Source: CAD feature listing. Evaluate the final solid. Frame: model axes, mm. A direction names the side the tool comes from. Round coordinates to 2 decimals unless told otherwise and drop trailing zeros. Loops run counter-clockwise (first coordinate to the right, second up) from the corner with the lowest first, then second, coordinate; pieces in that order, holes last. Notation, with made-up numbers: (-26, 19) - (-6, 19) arc R20 ccw to (-6, 51) - close; hole circle Ø2 at (88.5, 52.25). An arc over 180 degrees is marked (long way). One line per question, with ' | ' between items. Start each with the question number.
1. Cut plane A-A (x = 0). Return loops of the section in (y, z), then the cut area to 3 significant figures.
2. Pin query (flat end, axial travel): pin 1 (3 mm diameter, centred on x = -8.5, y = 35.5, fed in from +Z); pin 2 (1 mm diameter, centred on x = 0, y = 33, fed in from +Z); pin 3 (1.5 mm diameter, centred on x = 13, y = 9.5, fed in from +Z). Return the tip coordinate at first contact, or that it passes through.
3. Cut plane B-B (z = 19). Return loops of the section in (x, y), then the cut area to 3 significant figures.
4. Access query for faces 4 (the flat face through (9, 40, 39)), 5 (the flat face through (0, 48, 50)), 6 (the flat face through (5, 20, 10)). Directions: +Z, -Z, +X, -X, +Y, -Y. A direction counts if a zero-diameter tool reaches every point of the face in a straight line with its end or side. Return the directions, or none.
5. Cut plane D-D (z = 14). Return loops of the section in (x, y), then the cut area to 3 significant figures.
6. Cut plane C-C (y = 16). Return loops of the section in (x, z), then the cut area to 3 significant figures.
7. Ray query, line 1 (X direction, y = 26, z = 40); line 2 (Y direction, x = -6.5, z = 33.5); line 3 (Y direction, x = -3.5, z = 21.5). Return the intervals inside material, ascending.
8. Mould query, pull axis Y, two halves, no side actions, for faces 1 (the flat face through (-10, 20, 25)), 2 (the flat face through (-5, 6, 35)), 3 (the flat face through (-5, 0, 19)). Classes: pulls with the +Y half, pulls with the -Y half, needs draft (parallel to the pull), parting line crosses it, or undercut.
```python
from build123d import *

# Parameters (mm, degrees)
F1_DEPTH = 50
F3_W     = 30
F3_H     = 20
F4_DEPTH = 40
F5_DEPTH = 40


with BuildPart() as f1:
    # F0 (on Top) → F1 (new body)
    with BuildSketch(Plane.XY):
        with BuildLine():
            Line((-20, 40), (-20, 0))
            Line((-20, 0), (20, 0))
            Line((20, 0), (20, 40))
            ThreePointArc((20, 40), (0, 60), (-20, 40))
        make_face()
    extrude(amount=F1_DEPTH)

    # F3 (on face) → F4 (cut)
    with BuildSketch(Plane.XY.offset(50)):
        with Locations((5, 20)):
            Rectangle(F3_W, F3_H)
    extrude(amount=-F4_DEPTH, mode=Mode.SUBTRACT)

    # F2 (on face) → F5 (cut)
    with BuildSketch(Plane.XZ):
        Polygon((20, 50), (-20, 50), (20, 10), align=None)
    extrude(amount=-F5_DEPTH, mode=Mode.SUBTRACT)


solid = f1.part
```
Answers follow:
1) outline: (0, 0) - (60, 0) - (60, 50) - (40, 50) - (40, 30) - (30, 30) - (30, 10) - (10, 10) - (10, 30) - (0, 30) - close | area: 1,800 mm2
2) pin 1: stops at z = 40 | pin 2: stops at z = 30.5 | pin 3: stops at z = 17.75
3) outline: (-20, 0) - (11, 0) - (11, 10) - (-10, 10) - (-10, 30) - (11, 30) - (11, 40) - (20, 40) arc R20 ccw to (-20, 40) - close | area: 1,450 mm2
4) face 4: +Z, +X, -Y | face 5: +Z, +X, -X, +Y, -Y | face 6: +Z, +X
5) outline: (-20, 0) - (16, 0) - (16, 10) - (-10, 10) - (-10, 30) - (16, 30) - (16, 40) - (20, 40) arc R20 ccw to (-20, 40) - close | area: 1,550 mm2
6) outline: (-20, 0) - (20, 0) - (20, 10) - (-10, 10) - (-10, 40) - (-20, 50) - close | area: 750 mm2
7) line 1: x = -20 to -10 | line 2: y = 0 to 10, 30 to 58.91 | line 3: y = 0 to 10, 30 to 59.69
8) face 1: undercut | face 2: needs draft | face 3: pulls with the -Y half
